CAD build for the part. Positions are in the model's coordinates, mm. Round coordinates to 2 decimals unless told otherwise and drop trailing zeros. Write each loop counter-clockwise with the first axis right and the second up, starting at its lowest first coordinate (ties: lowest second). Pieces come first, ordered by that corner, then holes. Notation, with made-up numbers: (-21, 31) - (3, 31) arc R25 cw to (3, 47) - close; hole circle Ø5 at (49.25, 46.25). An arc over 180 degrees is marked (long way). Answer in a Markdown table with one row per item.
```python
from build123d import *

# Parameters (mm, degrees)
SKETCH2_W                = 19.932631385
SKETCH2_H                = 5.9
BOSS_EXTRUDE1_DEPTH      = 3
FILLET1_R                = 1
M3_CLEARANCE_HOLE1_D     = 3.4
M3_CLEARANCE_HOLE1_DEPTH = 16.5
M3_CLEARANCE_HOLE1_TIP   = 1.021463052


with BuildPart() as part:
    # Sketch2 → Boss-Extrude1 (new body)
    with BuildSketch(Plane.XY.offset(133.365661293)):
        with Locations((-21.255805031, 37.989811256)):
            Rectangle(SKETCH2_W, SKETCH2_H)
    extrude(amount=BOSS_EXTRUDE1_DEPTH)

    # Fillet1
    fillet1_edges = [part.edges().sort_by_distance(p)[0] for p in [
        (-31.222120723, 40.939811256, 134.865661293),
        (-11.289489338, 40.939811256, 134.865661293),
        (-11.289489338, 35.039811256, 134.865661293),
        (-31.222120723, 35.039811256, 134.865661293),
    ]]
    fillet(fillet1_edges, radius=FILLET1_R)

    # M3 Clearance Hole1
    with Locations(Plane.XY.offset(136.365661293)):
        with Locations((-28.757120723, 37.989811256), (-13.757120723, 37.989811256)):
            Hole(M3_CLEARANCE_HOLE1_D / 2, depth=M3_CLEARANCE_HOLE1_DEPTH)
            with Locations((0, 0, -(M3_CLEARANCE_HOLE1_DEPTH + M3_CLEARANCE_HOLE1_TIP / 2))):  # 118° drill point
                Cone(0, M3_CLEARANCE_HOLE1_D / 2, M3_CLEARANCE_HOLE1_TIP, mode=Mode.SUBTRACT)


solid = part.part
```
Q1. Saw through at C-C on z = 134.75. List the corners of the cut face in (x, y).
Computed:
| item | result |
|---|---|
| outline | (-31.22, 36.04) arc R1 ccw to (-30.22, 35.04) - (-12.29, 35.04) arc R1 ccw to (-11.29, 36.04) - (-11.29, 39.94) arc R1 ccw to (-12.29, 40.94) - (-30.22, 40.94) arc R1 ccw to (-31.22, 39.94) - close; hole circle Ø3.4 at (-28.76, 37.99); hole circle Ø3.4 at (-13.76, 37.99) |
Q2. Saw through at D-D on x = -28.75. List the corners of the cut face in (y, z), then the cut area to 3 significant figures.
Computed:
| item | result |
|---|---|
| outline | (35.04, 133.37) - (36.29, 133.37) - (36.29, 136.37) - (35.04, 136.37) - close; (39.69, 133.37) - (40.94, 133.37) - (40.94, 136.37) - (39.69, 136.37) - close |
| area | 7.50 mm2 |
Q3. Drill centre lines: line 1 (X direction, y = 38.1, z = 134.6); line 2 (X direction, y = 38.5, z = 135.45); line 3 (Y direction, x = -27.25, z = 135.9). Where is each one in solid material? Low to high.
Computed:
| item | result |
|---|---|
| line 1 | x = -31.22 to -30.45, -27.06 to -15.45, -12.06 to -11.29 |
| line 2 | x = -31.22 to -30.38, -27.14 to -15.38, -12.14 to -11.29 |
| line 3 | y = 35.04 to 37.2, 38.78 to 40.94 |
Q4. Pull direction Y, two halves, no side cores. Call faces 1 (the cylindrical face through (-30.937, 40.639, 134.887)), 2 (the cylindrical face through (-30.33, 37.34, 134.84)), 3 (the flat face through (-21, 35.04, 135)): released by +Y, released by -Y, zero draft, split by the parting line, or undercut.
Computed:
| item | result |
|---|---|
| face 1 | released by +Y |
| face 2 | undercut |
| face 3 | released by -Y |
Q5. Saw through at A-A on x = -13. List the corners of the cut face in (y, z), then the cut area to 3 significant figures.
Computed:
| item | result |
|---|---|
| outline | (35.04, 133.37) - (36.47, 133.37) - (36.47, 136.37) - (35.04, 136.37) - close; (39.51, 133.37) - (40.94, 133.37) - (40.94, 136.37) - (39.51, 136.37) - close |
| area | 8.57 mm2 |
Q6. Saw through at B-B on y = 37.1. List the corners of the cut face in (x, z).
Computed:
| item | result |
|---|---|
| outline | (-31.22, 133.37) - (-30.21, 133.37) - (-30.21, 136.37) - (-31.22, 136.37) - close; (-27.31, 133.37) - (-15.21, 133.37) - (-15.21, 136.37) - (-27.31, 136.37) - close; (-12.31, 133.37) - (-11.29, 133.37) - (-11.29, 136.37) - (-12.31, 136.37) - close |
